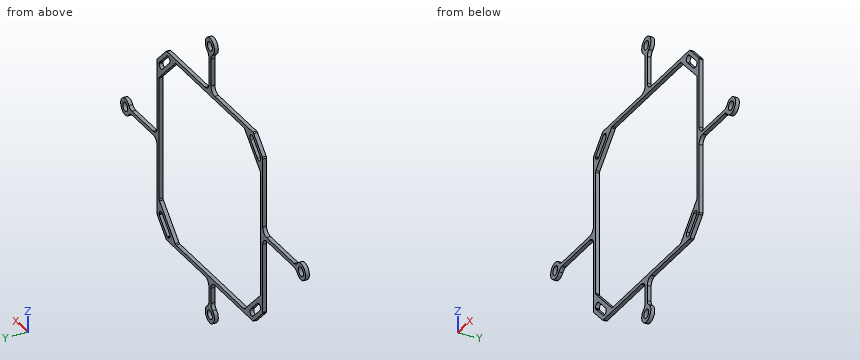
from build123d import *

# Parameters (mm, degrees)
SKETCH1_R           = 1.925
BOSS_EXTRUDE1_DEPTH = 1.65
FILLET4_R           = 3
FILLET3_R           = 1.5
FILLET5_R           = 1


with BuildPart() as part:
    # Sketch1 → Boss-Extrude1 (new body)
    with BuildSketch(Plane(origin=(0, 0, 0), x_dir=(1, 0, 0), z_dir=(0, 1, 0))):
        with BuildLine():
            Line((-41.448800006, 34.091704203), (-34.091704203, 41.448800006))
            Line((-34.091704203, 41.448800006), (-0.825, 41.448800006))
            Line((-0.825, 41.448800006), (-0.825, 52.97029458))
            ThreePointArc((-0.825, 52.97029458), (0, 60.023800006), (0.825, 52.97029458))
            Line((0.825, 52.97029458), (0.825, 41.448800006))
            Line((0.825, 41.448800006), (34.091704203, 41.448800006))
            Line((34.091704203, 41.448800006), (41.448800006, 34.091704203))
            Line((41.448800006, 34.091704203), (41.448800006, 0.825))
            Line((41.448800006, 0.825), (62.97029458, 0.825))
            ThreePointArc((62.97029458, 0.825), (70.023800006, 0), (62.97029458, -0.825))
            Line((62.97029458, -0.825), (41.448800006, -0.825))
            Line((41.448800006, -0.825), (41.448800006, -34.091704203))
            Line((41.448800006, -34.091704203), (34.091704203, -41.448800006))
            Line((34.091704203, -41.448800006), (0.825, -41.448800006))
            Line((0.825, -41.448800006), (0.825, -57.97029458))
            ThreePointArc((0.825, -57.97029458), (0, -65.023800006), (-0.825, -57.97029458))
            Line((-0.825, -57.97029458), (-0.825, -41.448800006))
            Line((-0.825, -41.448800006), (-34.091704203, -41.448800006))
            Line((-34.091704203, -41.448800006), (-41.448800006, -34.091704203))
            Line((-41.448800006, -34.091704203), (-41.448800006, -0.825))
            Line((-41.448800006, -0.825), (-67.97029458, -0.825))
            ThreePointArc((-67.97029458, -0.825), (-75.023800006, 0), (-67.97029458, 0.825))
            Line((-67.97029458, 0.825), (-41.448800006, 0.825))
            Line((-41.448800006, 0.825), (-41.448800006, 34.091704203))
        make_face()
        with Locations(Location((0, 56.448800006, 0), (0, 0, 270))):
            Circle(SKETCH1_R, mode=Mode.SUBTRACT)
        with Locations(Location((66.448800006, 0, 0), (0, 0, 90))):
            Circle(SKETCH1_R, mode=Mode.SUBTRACT)
        with Locations(Location((0, -61.448800006, 0), (0, 0, 270))):
            Circle(SKETCH1_R, mode=Mode.SUBTRACT)
        with Locations(Location((-71.448800006, 0, 0), (0, 0, 270))):
            Circle(SKETCH1_R, mode=Mode.SUBTRACT)
        Polygon((-39.798800006, 33.408251825), (-33.408251825, 39.798800006), (-29.292890359, 39.798800006), (-39.798800006, 29.292890359), align=None, mode=Mode.SUBTRACT)
        Polygon((-33.408251825, -39.798800006), (-29.292890359, -39.798800006), (-39.798800006, -29.292890359), (-39.798800006, -33.408251825), align=None, mode=Mode.SUBTRACT)
        Polygon((39.798800006, -33.408251825), (39.798800006, -29.292890359), (29.292890359, -39.798800006), (33.408251825, -39.798800006), align=None, mode=Mode.SUBTRACT)
        Polygon((33.408251825, 39.798800006), (39.798800006, 33.408251825), (39.798800006, 29.292890359), (29.292890359, 39.798800006), align=None, mode=Mode.SUBTRACT)
        Polygon((-39.798800006, 26.959437981), (-26.959437981, 39.798800006), (26.959437981, 39.798800006), (39.798800006, 26.959437981), (39.798800006, -26.959437981), (26.959437981, -39.798800006), (-26.959437981, -39.798800006), (-39.798800006, -26.959437981), align=None, mode=Mode.SUBTRACT)
    extrude(amount=BOSS_EXTRUDE1_DEPTH)

    # Fillet4
    fillet4_edges = [part.edges().sort_by_distance(p)[0] for p in [
        (-0.825, 0.825, -41.448800006),
        (-0.825, 0.825, -52.97029458),
        (0.825, 0.825, -52.97029458),
        (0.825, 0.825, -41.448800006),
        (41.448800006, 0.825, -0.825),
        (62.97029458, 0.825, -0.825),
        (62.97029458, 0.825, 0.825),
        (41.448800006, 0.825, 0.825),
        (0.825, 0.825, 41.448800006),
        (0.825, 0.825, 57.97029458),
        (-0.825, 0.825, 57.97029458),
        (-0.825, 0.825, 41.448800006),
        (-41.448800006, 0.825, 0.825),
        (-67.97029458, 0.825, 0.825),
        (-67.97029458, 0.825, -0.825),
        (-41.448800006, 0.825, -0.825),
    ]]
    fillet(fillet4_edges, radius=FILLET4_R)

    # Fillet3
    fillet3_edges = [part.edges().sort_by_distance(p)[0] for p in [
        (-29.292890359, 0.825, 39.798800006),
        (-39.798800006, 0.825, 29.292890359),
        (-39.798800006, 0.825, -29.292890359),
        (-29.292890359, 0.825, -39.798800006),
        (29.292890359, 0.825, -39.798800006),
        (39.798800006, 0.825, -29.292890359),
        (39.798800006, 0.825, 29.292890359),
        (29.292890359, 0.825, 39.798800006),
    ]]
    fillet(fillet3_edges, radius=FILLET3_R)

    # Fillet5
    fillet5_edges = [part.edges().sort_by_distance(p)[0] for p in [
        (-39.798800006, 0.825, -26.959437981),
        (-39.798800006, 0.825, 26.959437981),
        (-26.959437981, 0.825, 39.798800006),
        (26.959437981, 0.825, 39.798800006),
        (39.798800006, 0.825, 26.959437981),
        (39.798800006, 0.825, -26.959437981),
        (26.959437981, 0.825, -39.798800006),
        (-26.959437981, 0.825, -39.798800006),
        (-41.448800006, 0.825, -34.091704203),
        (-34.091704203, 0.825, -41.448800006),
        (34.091704203, 0.825, -41.448800006),
        (41.448800006, 0.825, -34.091704203),
        (41.448800006, 0.825, 34.091704203),
        (34.091704203, 0.825, 41.448800006),
        (-34.091704203, 0.825, 41.448800006),
        (-41.448800006, 0.825, 34.091704203),
    ]]
    fillet(fillet5_edges, radius=FILLET5_R)


solid = part.part
Model file for the job. Use its own axes, mm. Round coordinates to 2 decimals unless told otherwise and drop trailing zeros. Order: outer loops, then holes, each group sorted by start corner. A loop starts at its lowest first (then second) coordinate and runs counter-clockwise, first axis right, second up.
(1) Band-saw the part on C-C (y = 0.25). Give the number of separate pieces and of enclosed holes in the cut face, then the cut area to 3 significant figures.
(2) Band-saw the part on A-A (z = 22). List the corners of the cut face in (x, y), then the cut area to 4 significant figures.
(3) Band-saw the part on B-B (x = 15). List the corners of the cut face in (y, z), then the cut area to 4 significant figures.
(4) Pin check, flat tips, straight feed: pin 1 (0.5 mm diameter, centred on y = 0.5, z = -17.5, fed in from -X); pin 2 (5 mm diameter, centred on x = -34.5, z = 35, fed in from +Y); pin 3 (0.5 mm diameter, centred on y = 0.5, z = -11.5, fed in from +X); pin 4 (0.5 mm diameter, centred on x = -57, y = 1, fed in from -Z) (3 decimals). Stop position of each tip, or through.
(5) Drill centre lines: line 1 (Z direction, x = -12.5, y = 1.25); line 2 (Z direction, x = -2, y = 1.2). Where is each one in solid material? Low to high.
Verdict:
1. separate pieces: 1
1. enclosed holes: 9
1. area: 899 mm2
2. outline: (-41.45, 0) - (-39.8, 0) - (-39.8, 1.65) - (-41.45, 1.65) - close; (39.8, 0) - (41.45, 0) - (41.45, 1.65) - (39.8, 1.65) - close
2. area: 5.445 mm2
3. outline: (0, -41.45) - (1.65, -41.45) - (1.65, -39.8) - (0, -39.8) - close; (0, 39.8) - (1.65, 39.8) - (1.65, 41.45) - (0, 41.45) - close
3. area: 5.445 mm2
4. pin 1: stops at x = -41.45
4. pin 2: stops at y = 1.65
4. pin 3: stops at x = 41.45
4. pin 4: stops at z = -0.825
5. line 1: z = -41.45 to -39.8, 39.8 to 41.45
5. line 2: z = -59.41 to -53.48, -42.07 to -39.8, 39.8 to 42.07, 58.48 to 64.41
